Autodesk Fusion 360 part; units mm, degrees
sketch "Sketch1" plane through (0, 0, 0) normal (0, 1, 0) x (1, 0, 0)
  circle A0 centre (0, 0) radius 2.5
  circle A1 centre (12, 0) radius 2.5
  line L0 (-12, -12) -> (24, -12)
  line L1 (24, -12) -> (24, 10)
  line L2 (24, 10) -> (12, 32)
  line L3 (12, 32) -> (-12, 32)
  line L4 (-12, 32) -> (-12, -12)
  line L5 (0, 0) -> (0, 32) construction
  circle A2 centre (0, 20) radius 2.5
  line L6 (0, 0) -> (0, 20) construction
  point P0 (0, 10)
  dimension "d1" = 5
  dimension "d3" = 12
  dimension "d5" = 12
  dimension "d6" = 20
  dimension "d7" = 12
  dimension "d8" = 12
  dimension "d9" = 12
extrude "Extrude1" add sketch "Sketch1" along normal blind 20
fillet "Fillet1" radius 5 5 edges at (-12, 10, 12) (24, 10, 12) (-12, 10, -32) (12, 10, -32) (24, 10, -10)
sketch "Sketch2" plane through (0, 20, 0) normal (0, 1, 0) x (-1, 0, 0)
  arc A0 (-24, -8.725) -> (-23.3895, -11.1193) centre (-19, -8.725) ccw
  line L0 (-23.3895, -11.1193) -> (-13.4213, -29.3943)
  arc A1 (-13.4213, -29.3943) -> (-9.0318, -32) centre (-9.0318, -27) ccw
  line L1 (-9.0318, -32) -> (7, -32)
  arc A2 (7, -32) -> (12, -27) centre (7, -27) ccw
  line L2 (12, -27) -> (12, 7)
  arc A3 (12, 7) -> (7, 12) centre (7, 7) ccw
  line L3 (7, 12) -> (-19, 12)
  arc A4 (-19, 12) -> (-24, 7) centre (-19, 7) ccw
  line L4 (-24, 7) -> (-24, -8.725)
  circle A5 centre (0, -20) radius 2.5
  circle A6 centre (0, 0) radius 2.5
  circle A7 centre (-12, 0) radius 2.5
  line L5 (0, 0) -> (0, -20) construction
  line L6 (-3.75, 12) -> (3.75, 12)
  line L7 (3.75, 12) -> (3.75, -32)
  line L8 (3.75, -32) -> (-3.75, -32)
  line L9 (-3.75, -32) -> (-3.75, 12)
  dimension "d15" = 7.5
extrude "Extrude2" add sketch "Sketch2" along normal blind 2 contours L1 L3 L6 L7 L8 L9
chamfer "Chamfer1" distance 1 angle 45 2 edges at (3.75, 22, -10) (-3.75, 22, -10)
Geometry: final body of the model. Coordinates: model frame, mm. A direction names the side the tool comes from. Round coordinates to 2 decimals unless told otherwise and drop trailing zeros. Order: outer loops, then holes, each group sorted by start corner. A loop starts at its lowest first (then second) coordinate and runs counter-clockwise, first axis right, second up. Notation, with made-up numbers: (-18.75, 56) -> (20.25, 56) arc R18 ccw to (20.25, 88) -> close; hole circle Ø8 at (-20, -29). An arc over 180 degrees is marked (long way). Put each result on its own line as item: value. Start each with the question number.
Q1. First-contact query: pin 1 (4 mm diameter, centred on x = -6.5, z = -9.5, fed in from +Y); pin 2 (1 mm diameter, centred on y = 8.5, z = -9.5, fed in from +X). Flat tips, straight axial feed; report the tip coordinate or a pass-through.
Q2. Line query: probe 1 along Z at (x, y) = (0, 13); probe 2 along X at (y, z) = (14.5, 0); probe 3 along Z at (x, y) = (1, 5.5). Output: solid intervals per line, ascending.
Q3. Section B-B on x = 0. Return the cut outline in (y, z).
Q4. Section D-D on x = 12. Return the cut outline in (y, z), and give its area (3 significant figures).
Q5. Reachability of faces 1 (the flat face through (1, 11, -32)), 2 (the flat face through (3.75, 20.5, -10.3)), 3 (the flat face through (-8, 20, -10)) from +Z, -Z, +X, -X, +Y, -Y: full face, straight path, thin tool, end or side. Return the list, or none.
Q6. Section A-A on z = 0. Return the cut outline in (x, y), and give its area (3 significant figures).
Q7. Section C-C on y = 17.5. Return the cut outline in (x, z), and give its area (3 significant figures).
Ans:
1. pin 1: stops at y = 20
1. pin 2: stops at x = 23.99
2. probe 1: z = -32 to -22.5, -17.5 to -2.5, 2.5 to 12
2. probe 2: x = -12 to -2.5, 2.5 to 9.5, 14.5 to 24
2. probe 3: z = -32 to -22.29, -17.71 to -2.29, 2.29 to 12
3. outline: (0, -32) -> (22, -32) -> (22, -22.5) -> (0, -22.5) -> close; (0, -17.5) -> (22, -17.5) -> (22, -2.5) -> (0, -2.5) -> close; (0, 2.5) -> (22, 2.5) -> (22, 12) -> (0, 12) -> close
4. outline: (0, -31.02) -> (20, -31.02) -> (20, -2.5) -> (0, -2.5) -> close; (0, 2.5) -> (20, 2.5) -> (20, 12) -> (0, 12) -> close
4. area: 760 mm2
5. face 1: -Z, +X, -X, +Y, -Y
5. face 2: +Z, -Z, +X, +Y
5. face 3: +Z, -Z, -X, +Y
6. outline: (-12, 0) -> (-2.5, 0) -> (-2.5, 22) -> (-2.75, 22) -> (-3.75, 21) -> (-3.75, 20) -> (-12, 20) -> close; (2.5, 0) -> (9.5, 0) -> (9.5, 20) -> (3.75, 20) -> (3.75, 21) -> (2.75, 22) -> (2.5, 22) -> close; (14.5, 0) -> (24, 0) -> (24, 20) -> (14.5, 20) -> close
6. area: 524 mm2
7. outline: (-12, -27) arc R5 ccw to (-7, -32) -> (9.03, -32) arc R5 ccw to (13.42, -29.39) -> (23.39, -11.12) arc R5 ccw to (24, -8.73) -> (24, 7) arc R5 ccw to (19, 12) -> (-7, 12) arc R5 ccw to (-12, 7) -> close; hole circle Ø5 at (0, -20); hole circle Ø5 at (0, 0); hole circle Ø5 at (12, 0)
7. area: 1,380 mm2
